from build123d import *

# Parameters (mm, degrees)
F0_W     = 15.875
F0_H     = 101.6
F0_W_2   = 3.81
F1_DEPTH = 3.81
F2_DEPTH = 3.81


with BuildPart() as f1:
    # F0 (on Front) → F1 (new body)
    with BuildSketch(Plane.XZ):
        with Locations((-68.512963, -50.470196)):
            Rectangle(F0_W, F0_H)
        with Locations((-37.397963, -50.470196)):
            Rectangle(F0_W, F0_H)
        with Locations((-58.670463, -50.470196)):
            Rectangle(F0_W_2, F0_H)
        with Locations((-47.240463, -50.470196)):
            Rectangle(F0_W_2, F0_H)
        with Locations((-27.555463, -50.470196)):
            Rectangle(F0_W_2, F0_H)
        with Locations((-78.355463, -50.470196)):
            Rectangle(F0_W_2, F0_H)
        Polygon((-52.955463, -4.750196), (-56.765463, 0.329804), (-56.765463, -101.270196), (-49.145463, -101.270196), (-49.145463, 0.329804), align=None)
    extrude(amount=F1_DEPTH)

    # F0 (on Front) → F2 (join)
    with BuildSketch(Plane.XZ):
        with Locations((-58.670463, -50.470196)):
            Rectangle(F0_W_2, F0_H)
        with Locations((-47.240463, -50.470196)):
            Rectangle(F0_W_2, F0_H)
        with Locations((-27.555463, -50.470196)):
            Rectangle(F0_W_2, F0_H)
        with Locations((-78.355463, -50.470196)):
            Rectangle(F0_W_2, F0_H)
    extrude(amount=-F2_DEPTH)


solid = f1.part
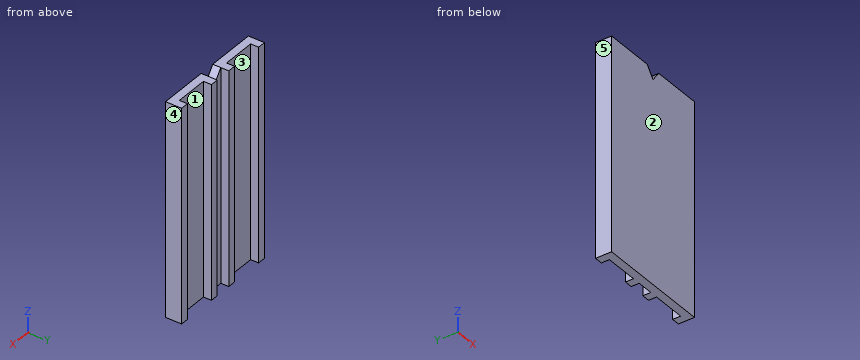
The listing builds one solid part. Answer for the finished solid, in the listing's coordinates (mm). Face numbers are marked on the shaded views. A direction names the side the tool comes from. Give positions to 0.01 mm unless a question says otherwise; leave off trailing zeros. Write each loop counter-clockwise with the first axis right and the second up, starting at its lowest first coordinate (ties: lowest second). Pieces come first, ordered by that corner, then holes. Notation, with made-up numbers: (-1.5, 8) -> (15.5, 8) arc R20 ccw to (15.5, 13) -> close; hole circle Ø11 at (-14.75, 77). An arc over 180 degrees is marked (long way). Use a Markdown table: item, result.
(1) Determine the mould class of the marked faces 3, 4 and 5 for opening direction X: released by +X, released by -X, zero draft, split by the parting line, or undercut.
Return value:
| item | result |
|---|---|
| face 3 | undercut |
| face 4 | released by +X |
| face 5 | released by -X |
(2) For the marked faces 1 and 2, determine the directions among +Z, -Z, +X, -X, +Y, -Y from which every point of the face is accessible in a straight line to the end or side of a thin tool.
Return value:
| item | result |
|---|---|
| face 1 | +Z, -Z, +Y |
| face 2 | +Z, -Z, +X, -X, -Y |
(3) Section A-A, the plane y = 1 is taken. Determine the outline of the cut face in (x, z).
Return value:
| item | result |
|---|---|
| outline | (-80.26, -101.27) -> (-76.45, -101.27) -> (-76.45, 0.33) -> (-80.26, 0.33) -> close; (-60.58, -101.27) -> (-56.77, -101.27) -> (-56.77, 0.33) -> (-60.58, 0.33) -> close; (-49.15, -101.27) -> (-45.34, -101.27) -> (-45.34, 0.33) -> (-49.15, 0.33) -> close; (-29.46, -101.27) -> (-25.65, -101.27) -> (-25.65, 0.33) -> (-29.46, 0.33) -> close |
(4) Section C-C, the plane x = -70.5 is taken. Determine the outline of the cut face in (y, z).
Return value:
| item | result |
|---|---|
| outline | (-3.81, -101.27) -> (0, -101.27) -> (0, 0.33) -> (-3.81, 0.33) -> close |
(5) Section B-B, the plane z = -59 is taken. Determine the outline of the cut face in (x, y).
Return value:
| item | result |
|---|---|
| outline | (-80.26, -3.81) -> (-25.65, -3.81) -> (-25.65, 3.81) -> (-29.46, 3.81) -> (-29.46, 0) -> (-45.34, 0) -> (-45.34, 3.81) -> (-49.15, 3.81) -> (-49.15, 0) -> (-56.77, 0) -> (-56.77, 3.81) -> (-60.58, 3.81) -> (-60.58, 0) -> (-76.45, 0) -> (-76.45, 3.81) -> (-80.26, 3.81) -> close |
(6) Find the intervals of material crossed by probe 1 along X at (y, z) = (0.75, -67.5); probe 2 along Y at (x, z) = (-63, -28.5), in increasing order. Write a range as from..to.
Return value:
| item | result |
|---|---|
| probe 1 | -80.26..-76.45, -60.58..-56.77, -49.15..-45.34, -29.46..-25.65 |
| probe 2 | -3.81..0 |
(7) Flat-ended cylindrical pins translate along their axes: P1, Ø1.5, axis at x = -70, y = 0.5, coming from the +Z side; P2, Ø5, axis at x = -67, z = -29, coming from the +Y side. Find the tip coordinate at first contact, or state that the pin passes through.
Return value:
| item | result |
|---|---|
| P1 | z = 0.33 |
| P2 | y = 0 |
